```python
from build123d import *

# Parameters (mm, degrees)
BOSS_EXTRUDE1_DEPTH = 1.6
CUT_EXTRUDE1_REACH  = 134.452
SKETCH3_W           = 5.911971619
SKETCH3_H           = 1
BOSS_EXTRUDE2_DEPTH = 1.6
BOSS_EXTRUDE3_DEPTH = 1.6
FILLET2_R           = 1
SKETCH6_R           = 1.6
CUT_EXTRUDE2_DEPTH  = 133.452104551
BOSS_EXTRUDE4_DEPTH = 1.6
FILLET3_R           = 3


with BuildPart() as part:
    # Sketch1 → Boss-Extrude1 (new body)
    with BuildSketch(Plane.XY):
        with BuildLine():
            Line((-25, 2), (-25, 0))
            Line((-25, 0), (-82, 0))
            Line((-82, 0), (-82, 2))
            Line((-82, 2), (-85, 2))
            Line((-85, 2), (-85, 0))
            Line((-85, 0), (-97, 0))
            Line((-97, 0), (-97, -3.2))
            Line((-97, -3.2), (-103, -3.2))
            Line((-103, -3.2), (-103, 0))
            Line((-103, 0), (-115, 0))
            Line((-115, 0), (-115, 2))
            Line((-115, 2), (-118, 2))
            Line((-118, 2), (-118, 0))
            Line((-118, 0), (-126, 0))
            ThreePointArc((-126, 0), (-128.982873168, -2.679894289), (-126.636556491, -5.931688223))
            Line((-126.636556491, -5.931688223), (-25, -28))
            Line((-25, -28), (-25, -30))
            Line((-25, -30), (-21, -30))
            Line((-21, -30), (-21, 2))
            Line((-21, 2), (-25, 2))
        make_face()
        Polygon((-32, -21.363586453), (-64.968742205, -14.205094401), (-32, -7.046602348), align=None, mode=Mode.SUBTRACT)
        Polygon((-69.038028381, -5), (-36.712857451, -5), (-69.038028381, -12.018753635), align=None, mode=Mode.SUBTRACT)
        Polygon((-72.038028381, -5), (-72.038028381, -12.67014264), (-107.363199311, -5), align=None, mode=Mode.SUBTRACT)
    extrude(amount=BOSS_EXTRUDE1_DEPTH)

    # Sketch2 → Cut-Extrude1 (cut, up to next)
    with BuildSketch(Plane.XY.offset(1.6), mode=Mode.PRIVATE) as cut_extrude1_sk1:
        Polygon((-122.05, -5), (-114.05, -5), (-114.05, -8.664603056), (-122.05, -6.927565711), align=None)
    cut_extrude1_tool1 = extrude(cut_extrude1_sk1.sketch, amount=-CUT_EXTRUDE1_REACH, mode=Mode.PRIVATE) & part.part
    add(cut_extrude1_tool1.solids().sort_by_distance((-117.635841, -6.443005, 1.6))[0], mode=Mode.SUBTRACT)

    # Sketch3 → Boss-Extrude2 (add)
    with BuildSketch(Plane.XY.offset(1.6)):
        with Locations((-74.99401419, -5.5)):
            Rectangle(SKETCH3_W, SKETCH3_H)
        with Locations((-88.90598581, -5.5)):
            Rectangle(SKETCH3_W, SKETCH3_H)
    extrude(amount=-BOSS_EXTRUDE2_DEPTH)

    # Sketch4 → Boss-Extrude3 (add)
    with BuildSketch(Plane.XY.offset(1.6)):
        Polygon((-107.363199311, -5), (-94, -5), (-94, -7.901547031), align=None)
    extrude(amount=-BOSS_EXTRUDE3_DEPTH)

    # Fillet2
    fillet2_edges = [part.edges().sort_by_distance(p)[0] for p in [
        (-64.968742205, -14.205094401, 0.8),
        (-69.038028381, -12.018753635, 0.8),
        (-72.038028381, -12.67014264, 0.8),
        (-69.038028381, -5, 0.8),
        (-36.712857451, -5, 0.8),
        (-32, -7.046602348, 0.8),
        (-32, -21.363586453, 0.8),
        (-122.05, -5, 0.8),
        (-114.05, -5, 0.8),
        (-85.95, -5, 0.8),
        (-77.95, -5, 0.8),
        (-72.038028381, -6, 0.8),
        (-91.861971619, -5, 0.8),
        (-94, -7.901547031, 0.8),
        (-94, -5, 0.8),
    ]]
    fillet(fillet2_edges, radius=FILLET2_R - 0.0001)  # a hair under: the kernel refuses the full size

    # Sketch6 → Cut-Extrude2 (cut, through all)
    with BuildSketch(Plane.XY.offset(1.6)):
        with Locations((-26.5, -14)):
            Circle(SKETCH6_R)
    extrude(amount=-CUT_EXTRUDE2_DEPTH, mode=Mode.SUBTRACT)

    # Sketch5 → Boss-Extrude4 (add)
    with BuildSketch(Plane.XY.offset(1.6)):
        with BuildLine():
            Line((-72.502917062, -17.685707385), (-88.939743507, -111.308320091))
            ThreePointArc((-88.939743507, -111.308320091), (-86.37296732, -115.756988254), (-81.542598068, -114.011559564))
            Line((-81.542598068, -114.011559564), (-31.5, -28))
            Line((-31.5, -28), (-25, -28))
            Line((-25, -28), (-34.87966647, -25.854831299))
            Line((-34.87966647, -25.854831299), (-82.18159936, -107.155826358))
            ThreePointArc((-82.18159936, -107.155826358), (-83.389191673, -107.59218353), (-84.03088572, -106.48001649))
            Line((-84.03088572, -106.48001649), (-68.590867503, -18.535129407))
            Line((-68.590867503, -18.535129407), (-72.502917062, -17.685707385))
        make_face()
    extrude(amount=-BOSS_EXTRUDE4_DEPTH)

    # Fillet3
    fillet3_edges = [part.edges().sort_by_distance(p)[0] for p in [
        (-72.502917062, -17.685707385, 0.8),
        (-68.590867503, -18.535129407, 0.8),
        (-34.87966647, -25.854831299, 0.8),
        (-31.5, -28, 0.8),
    ]]
    fillet(fillet3_edges, radius=FILLET3_R)


solid = part.part
```
Verification items for the finished model (mm, model axes). A direction names the side the tool comes from. Give positions to 0.01 mm unless a question says otherwise; leave off trailing zeros. Loops run counter-clockwise (first coordinate to the right, second up) from the corner with the lowest first, then second, coordinate; pieces in that order, holes last.
1. Set-up check for faces 1 (the flat face through (-71, -31, 0)), 2 (the flat face through (-80.86, -65.28, 0.81)), 3 (the flat face through (-56.668, -9.333, 0.789)): record each of +Z, -Z, +X, -X, +Y, -Y from which the full face is reachable in a straight line by a thin tool's end or side.
2. Section check B-B, the plane y = -69. Enter the section's corners in (x, z), then the cut area to 3 significant figures.
3. Section check C-C, the plane z = 0.25. Count the separate pieces of the cut face and the enclosed holes in it, then the cut area to 3 significant figures.
4. Section check A-A, the plane x = -26.5. Enter the section's corners in (y, z).
5. Mould release check, pull along Y, two halves, no side actions. Record for faces 4 (the flat face through (-71, -31, 1.6)), 5 (the cylindrical face through (-129, -3, 1)), 6 (the flat face through (-47.03, -10.31, 0.79)), 7 (the cylindrical face through (-27.68, -12.92, 0.81)): released by +Y, released by -Y, zero draft, split by the parting line, or undercut.
6. Section check D-D, the plane x = -110.5. Enter the section's corners in (y, z), then the cut area to 3 significant figures.
7. Thickness scan on line 1 (Y direction, x = -26.5, z = 0.6); line 2 (Y direction, x = -52, z = 1.3); line 3 (Y direction, x = -50, z = 0.95). Record the ranges inside material, lowest first.
8. Go/stop test with flat-tipped pins: pin 1 Ø0.5 at (x, z) = (-75, 1) entering from -Y; pin 2 Ø0.5 at (y, z) = (-29, 1) entering from -X; pin 3 Ø0.8 at (x, z) = (-119, 1) entering from -Y. Record where each tip stops, or that it passes through.
Geometry says:
1. face 1: -Z, +X, -X, +Y, -Y
1. face 2: +Z, -Z, -X
1. face 3: +Z, -Z
2. outline: (-81.51, 0) - (-77.45, 0) - (-77.45, 1.6) - (-81.51, 1.6) - close; (-59.98, 0) - (-55.35, 0) - (-55.35, 1.6) - (-59.98, 1.6) - close
2. area: 13.9 mm2
3. separate pieces: 1
3. enclosed holes: 5
3. area: 2,210 mm2
4. outline: (-28, 0) - (-15.6, 0) - (-15.6, 1.6) - (-28, 1.6) - close; (-12.4, 0) - (0, 0) - (0, 1.6) - (-12.4, 1.6) - close
5. face 4: zero draft
5. face 5: split by the parting line
5. face 6: undercut
5. face 7: undercut
6. outline: (-9.44, 0) - (0, 0) - (0, 1.6) - (-9.44, 1.6) - close
6. area: 15.1 mm2
7. line 1: y = -28 to -15.6, -12.4 to 0
7. line 2: y = -63.23 to -55.28, -22.14 to -17.02, -11.39 to -8.32, -5 to 0
7. line 3: y = -59.8 to -51.84, -22.57 to -17.46, -10.95 to -7.89, -5 to 0
8. pin 1: stops at y = -103.2
8. pin 2: stops at x = -74.53
8. pin 3: stops at y = -5
